Geometry: final body of the model. Coordinates: model frame, mm. A direction names the side the tool comes from. Coordinates: 2 decimals unless noted, no trailing zeros. Write each loop counter-clockwise with the first axis right and the second up, starting at its lowest first coordinate (ties: lowest second). Pieces come first, ordered by that corner, then holes. Notation, with made-up numbers: (5, -34.5) - (19, -34.5) arc R36 cw to (19, 1.5) - close; hole circle Ø8 at (-38.5, -29). An arc over 180 degrees is marked (long way). Answer as a JSON object with one key per item and string values. Group by question number.
Item 1: Section A-A on y = 7. Return loops of the section in (x, z).
Item 2: Line query: line 1 along X through (y, z) = (7, 0); line 2 along Z through (x, y) = (-154.5, -4); line 3 along X through (y, z) = (18, -3). Output: solid intervals per line, ascending. Write a range as from..to.
Item 3: First-contact query: pin 1 Ø1.5 at (x, y) = (-131, 6) entering from +Z; pin 2 Ø3 at (y, z) = (-8, 31.5) entering from +X; pin 3 Ø3 at (x, y) = (32.5, 12) entering from +Z; pin 4 Ø16 at (x, z) = (211.06, 0) entering from +Y. Flat tips, straight axial feed; report the tip coordinate or a pass-through.
Item 4: Section B-B on x = -61.5. Return loops of the section in (y, z).
Item 5: Set-up query: faces 1 (the flat face through (-135.654, 0, 35)), 2 (the flat face through (-115.9, -12.5, 39.8)), 3 (the flat face through (-95.654, 0, 35)), 4 (the flat face through (-115.9, 12.5, 39.8)). Return all of +Z, -Z, +X, -X, +Y, -Y with unobstructed straight access to the full face (end or side cutting, diameter ignored); none if empty.
```python
from build123d import *

# Parameters (mm, degrees)
F0_W     = 20
F0_H     = 20
F1_DEPTH = 20
F2_DEPTH = 12.5
F3_D     = 20
F3_DEPTH = 20.001
F4_D     = 20


with BuildPart() as f1:
    # F0 (on Front) → F1 (new body, symmetric)
    with BuildSketch(Plane.XZ):
        with BuildLine():
            ThreePointArc((-115.6540289521, -20), (-101.5118933284, -14.1421356237), (-95.6540289521, 0))
            Line((-95.6540289521, 0), (-115.6540289521, 0))
            Line((-115.6540289521, 0), (-135.6540289521, 0))
            ThreePointArc((-135.6540289521, 0), (-129.7961645759, -14.1421356237), (-115.6540289521, -20))
        make_face()
        with BuildLine():
            Line((-95.6540289521, 20), (-95.6540289521, 0))
            ThreePointArc((-95.6540289521, 0), (-101.5118933284, -14.1421356237), (-115.6540289521, -20))
            Line((-115.6540289521, -20), (211.0609319716, -20))
            ThreePointArc((211.0609319716, -20), (231.0609319716, 0), (211.0609319716, 20))
            Line((211.0609319716, 20), (-95.6540289521, 20))
        make_face()
        with Locations((-105.6540289521, 10)):
            Rectangle(F0_W, F0_H)
        with Locations((-125.6540289521, 10)):
            Rectangle(F0_W, F0_H)
        with BuildLine():
            Line((-238.9390680284, -20), (-115.6540289521, -20))
            ThreePointArc((-115.6540289521, -20), (-129.7961645759, -14.1421356237), (-135.6540289521, 0))
            Line((-135.6540289521, 0), (-135.6540289521, 20))
            Line((-135.6540289521, 20), (-238.9390680284, 20))
            ThreePointArc((-238.9390680284, 20), (-258.9390680284, 0), (-238.9390680284, -20))
        make_face()
    extrude(amount=F1_DEPTH, both=True)

    # F0 (on Front) → F2 (join, symmetric)
    with BuildSketch(Plane.XZ):
        with BuildLine():
            ThreePointArc((-115.6540289521, -20), (-101.5118933284, -14.1421356237), (-95.6540289521, 0))
            Line((-95.6540289521, 0), (-115.6540289521, 0))
            Line((-115.6540289521, 0), (-135.6540289521, 0))
            ThreePointArc((-135.6540289521, 0), (-129.7961645759, -14.1421356237), (-115.6540289521, -20))
        make_face()
        with BuildLine():
            Line((-95.6540289521, 20), (-95.6540289521, 0))
            ThreePointArc((-95.6540289521, 0), (-101.5118933284, -14.1421356237), (-115.6540289521, -20))
            Line((-115.6540289521, -20), (211.0609319716, -20))
            ThreePointArc((211.0609319716, -20), (231.0609319716, 0), (211.0609319716, 20))
            Line((211.0609319716, 20), (-95.6540289521, 20))
        make_face()
        with Locations((-105.6540289521, 10)):
            Rectangle(F0_W, F0_H)
        with Locations((-125.6540289521, 10)):
            Rectangle(F0_W, F0_H)
        with BuildLine():
            Line((-238.9390680284, -20), (-115.6540289521, -20))
            ThreePointArc((-115.6540289521, -20), (-129.7961645759, -14.1421356237), (-135.6540289521, 0))
            Line((-135.6540289521, 0), (-135.6540289521, 20))
            Line((-135.6540289521, 20), (-238.9390680284, 20))
            ThreePointArc((-238.9390680284, 20), (-258.9390680284, 0), (-238.9390680284, -20))
        make_face()
        with BuildLine():
            Line((-115.6540289521, 20), (-95.6540289521, 20))
            Line((-95.6540289521, 20), (-95.6540289521, 50.1140356064))
            ThreePointArc((-95.6540289521, 50.1140356064), (-115.6540289521, 70.1140356064), (-135.6540289521, 50.1140356064))
            Line((-135.6540289521, 50.1140356064), (-135.6540289521, 20))
            Line((-135.6540289521, 20), (-115.6540289521, 20))
        make_face()
    extrude(amount=F2_DEPTH, both=True)

    # F3 (through all, one way)
    with BuildSketch(Plane(origin=(0, 0, 0), x_dir=(1, 0, 0), z_dir=(0, 1, 0))):
        with Locations((211.0609319716, 0), (-115.6540289521, -50.1140356064)):
            Circle(F3_D / 2)
    extrude(amount=-F3_DEPTH, mode=Mode.SUBTRACT)

    # F4 (through all)
    with Locations(Plane.XZ):
        with Locations((-115.6540289521, 50.1140356064), (211.0609319716, 0)):
            Hole(F4_D / 2)


solid = f1.part
```
Checks:
{
 "1": {"outline": "(-238.94, -20) - (211.06, -20) arc R20 ccw to (211.06, 20) - (-95.65, 20) - (-95.65, 50.11) arc R20 ccw to (-135.65, 50.11) - (-135.65, 20) - (-238.94, 20) arc R20 ccw to start; hole circle Ø20 at (-115.65, 50.11); hole circle Ø20 at (211.06, 0)"},
 "2": {"line 1": "-258.94..201.06, 221.06..231.06", "line 2": "-20..20", "line 3": "-258.71..201.52, 220.6..230.83"},
 "3": {"pin 1": "z = 63.79", "pin 2": "x = -95.65", "pin 3": "z = 20", "pin 4": "through"},
 "4": {"outline": "(-20, -20) - (20, -20) - (20, 20) - (-20, 20) - close"},
 "5": {"face 1": "+Z, -X, +Y, -Y", "face 2": "+Z, +X, -X, -Y", "face 3": "+Z, +X, +Y, -Y", "face 4": "+Z, +X, -X, +Y"}
}
